Autodesk Inventor part; units mm, degrees
ref_plane "YZ Plane" through (0, 0, 0) normal (1, 0, 0) x (0, 1, 0)
ref_plane "XZ Plane" through (0, 0, 0) normal (0, 1, 0) x (-1, 0, 0)
ref_plane "XY Plane" through (0, 0, 0) normal (0, 0, 1) x (1, 0, 0)
sketch "스케치1" plane through (0, 0, 0) normal (0, 0, 1) x (1, 0, 0)
  line L0 (-28, 61.1) -> (28, 61.1)
  line L1 (28, 61.1) -> (28, -5.1)
  line L2 (28, -5.1) -> (-28, -5.1)
  line L3 (-28, -5.1) -> (-28, 61.1)
  point P0 (0, 0)
  dimension "d0" = 66.2
  dimension "d2" = 5.1
  dimension "d8" = 28
  dimension "d9" = 28
extrude "돌출1" add sketch "스케치1" along normal blind 4
sketch "스케치2" plane through (0, 0, 4) normal (0, 0, 1) x (1, 0, 0)
  line L0 (-2, 48) -> (-2, 6)
  line L1 (-32, 48) -> (-7.5, 48)
  line L2 (-2, 48) -> (4.5, 48)
  line L3 (16.5, 6) -> (16.5, 48)
  line L4 (10, 48) -> (16.5, 48)
  line L5 (10, 48) -> (10, 6)
  line L6 (10, 6) -> (16.5, 6)
  circle A0 centre (13, 45) radius 1.6
  circle A1 centre (13, 9) radius 1.6
  line L7 (28.5, 6) -> (28.5, 48)
  line L8 (22, 48) -> (28.5, 48)
  line L9 (22, 48) -> (22, 6)
  line L10 (22, 6) -> (28.5, 6)
  circle A2 centre (25, 45) radius 1.6
  circle A3 centre (25, 9) radius 1.6
  line L11 (-7.5, 6) -> (-7.5, 48)
  line L12 (-32, 48) -> (-7.5, 48)
  line L13 (-32, 48) -> (-32, 52)
  line L14 (-38, 52) -> (-32, 52)
  line L15 (-38, 2) -> (-38, 52)
  line L16 (-38, 2) -> (-32, 2)
  line L17 (-32, 2) -> (-32, 6)
  line L18 (-32, 6) -> (-7.5, 6)
  circle A4 centre (-35, 45) radius 1.6
  circle A5 centre (-35, 9) radius 1.6
  circle A6 centre (-23, 45) radius 1.6
  circle A7 centre (-23, 9) radius 1.6
  circle A8 centre (-11, 45) radius 1.6
  circle A9 centre (-11, 9) radius 1.6
  line L19 (-2, 6) -> (4.5, 6)
  circle A10 centre (1, 45) radius 1.6
  circle A11 centre (1, 9) radius 1.6
  line L20 (-2, 48) -> (0, 48)
  line L21 (0, 48) -> (0, 6)
  point P0 (0, 0)
  point P1 (-13, 26)
  dimension "d7" = 2
extrude "돌출2" cut sketch "스케치2" against normal up to surface (4 mm away) contours L21 A10 | A10 L21 | L21 A11 | A11 L21 | A0 | A1 | A2 | A3 | A6 | A7 | A8 | A9
sketch "스케치3" plane through (0, 0, 4) normal (0, 0, 1) x (1, 0, 0)
  circle A0 centre (-23, 45) radius 1.6
  circle A1 centre (-11, 45) radius 1.6
  circle A2 centre (-11, 9) radius 1.6
  circle A3 centre (25, 9) radius 1.6
  circle A4 centre (13, 45) radius 1.6
  circle A5 centre (1, 9) radius 1.6
  circle A6 centre (1, 45) radius 1.6
  circle A7 centre (13, 9) radius 1.6
  circle A8 centre (25, 45) radius 1.6
  circle A9 centre (-23, 9) radius 1.6
  line L0 (28, 61.1) -> (-28, 61.1)
  line L1 (-28, 61.1) -> (-28, -5.1)
  line L2 (-28, -5.1) -> (28, -5.1)
  line L3 (28, -5.1) -> (28, 61.1)
  line L4 (-23, 45) -> (-23, 9)
  line L5 (-23, 27) -> (-28, 27)
  line L6 (-28, -5.1) -> (-28, 61.1)
  circle A10 centre (-28, 27) radius 5
  point P0 (0, 0)
  dimension "d12" = 18
  dimension "d15" = 10
extrude "돌출3" cut sketch "스케치3" against normal blind 4 contours A10 L5 L1 | L1 A10 | L5 A10 L1
sketch "스케치4" plane through (0, 0, 4) normal (0, 0, 1) x (1, 0, 0)
  arc A0 (-28, 22) -> (-28, 32) centre (-28, 27) ccw
  line L0 (-28, 22) -> (-28, -5.1)
  line L1 (-28, -5.1) -> (28, -5.1)
  line L2 (28, -5.1) -> (28, 61.1)
  line L3 (28, 61.1) -> (-28, 61.1)
  line L4 (-28, 61.1) -> (-28, 32)
  circle A1 centre (-23, 9) radius 1.6
  circle A2 centre (25, 45) radius 1.6
  circle A3 centre (13, 9) radius 1.6
  circle A4 centre (1, 45) radius 1.6
  circle A5 centre (1, 9) radius 1.6
  circle A6 centre (13, 45) radius 1.6
  circle A7 centre (25, 9) radius 1.6
  circle A8 centre (-11, 9) radius 1.6
  circle A9 centre (-11, 45) radius 1.6
  circle A10 centre (-23, 45) radius 1.6
  circle A11 centre (-18, -2.6) radius 1.6
  circle A12 centre (-8, -2.6) radius 1.6
  circle A13 centre (8, -2.6) radius 1.6
  circle A14 centre (18, -2.6) radius 1.6
  point P0 (0, 0)
  dimension "d16" = 3.2
  dimension "d17" = 3.2
  dimension "d18" = 3.2
  dimension "d19" = 3.2
  dimension "d20" = 2.5
  dimension "d21" = 2.5
  dimension "d22" = 2.5
  dimension "d23" = 2.5
  dimension "d24" = 10
  dimension "d25" = 20
  dimension "d26" = 10
  dimension "d27" = 20
extrude "돌출4" cut sketch "스케치4" against normal up to surface (4 mm away) contours A11 | A12 | A13 | A14
sketch "스케치5" plane through (0, 0, 4) normal (0, 0, 1) x (1, 0, 0)
  circle A0 centre (8, -2.6) radius 1.6
  circle A1 centre (18, -2.6) radius 1.6
  circle A2 centre (-8, -2.6) radius 1.6
  circle A3 centre (-18, -2.6) radius 1.6
  arc A4 (-28, 22) -> (-28, 32) centre (-28, 27) ccw
  line L0 (-28, 22) -> (-28, -5.1)
  line L1 (-28, -5.1) -> (28, -5.1)
  line L2 (28, -5.1) -> (28, 61.1)
  line L3 (28, 61.1) -> (-28, 61.1)
  line L4 (-28, 61.1) -> (-28, 32)
  circle A5 centre (-23, 9) radius 1.6
  circle A6 centre (25, 45) radius 1.6
  circle A7 centre (13, 9) radius 1.6
  circle A8 centre (1, 45) radius 1.6
  circle A9 centre (1, 9) radius 1.6
  circle A10 centre (13, 45) radius 1.6
  circle A11 centre (25, 9) radius 1.6
  circle A12 centre (-11, 9) radius 1.6
  circle A13 centre (-11, 45) radius 1.6
  circle A14 centre (-23, 45) radius 1.6
  circle A15 centre (-18, 56.6) radius 1.6
  circle A16 centre (-8, 56.6) radius 1.6
  circle A17 centre (8, 56.6) radius 1.6
  circle A18 centre (18, 56.6) radius 1.6
  point P0 (0, 0)
  dimension "d30" = 3.2
  dimension "d31" = 3.2
  dimension "d32" = 3.2
  dimension "d33" = 3.2
  dimension "d34" = 4.5
  dimension "d35" = 4.5
  dimension "d36" = 4.5
  dimension "d37" = 4.5
  dimension "d38" = 10
  dimension "d39" = 20
  dimension "d40" = 10
  dimension "d41" = 20
extrude "돌출5" cut sketch "스케치5" against normal up to surface (4 mm away) contours A15 | A16 | A17 | A18
fillet "모깎기1" radius 3 1 edges at (-28, 61.1, 2)
chamfer "모따기1" distance 1.5 angle 45 8 edges at (-19.6, 56.6, 4) (-9.6, 56.6, 4) (6.4, 56.6, 4) (16.4, 56.6, 4) (-19.6, 56.6, 0) (-9.6, 56.6, 0) (6.4, 56.6, 0) (16.4, 56.6, 0)
chamfer "모따기2" distance 1.5 angle 45 10 edges at (23.4, 45, 4) (11.4, 45, 4) (-0.6, 45, 4) (-12.6, 45, 4) (-24.6, 45, 4) (-24.6, 9, 4) (-12.6, 9, 4) (-0.6, 9, 4) (11.4, 9, 4) (23.4, 9, 4)
properties part number "J1J2_Side" material "알루미늄 6061"
The listing builds one solid part. Answer for the finished solid, in the listing's coordinates (mm). Coordinates: 2 decimals unless noted, no trailing zeros. Loops run counter-clockwise (first coordinate to the right, second up) from the corner with the lowest first, then second, coordinate; pieces in that order, holes last. Notation, with made-up numbers: (36, 30) -> (64, 30) arc R15 ccw to (64, 55) -> close; hole circle Ø2 at (27, 4.25). An arc over 180 degrees is marked (long way). Answer in a Markdown table with one row per item. Add a question column.
1. The part is cut by section B-B, the plane x = 13. Write down the section's boundary in (y, z).
2. Flat-ended cylindrical pins translate along their axes: P1, Ø4, axis at x = -18, y = 56.6, coming from the +Z side; P2, Ø2, axis at x = 18, y = 27, coming from the -Z side; P3, Ø1.9, axis at x = -8, y = 56.6, coming from the +Z side; P4, Ø5, axis at x = -23, y = 9, coming from the +Z side. Find the tip coordinate at first contact, or state that the pin passes through.
3. Consider line 1 (Y direction, x = -11, z = 1.1); line 2 (Y direction, x = 8, z = 1.9); line 3 (X direction, y = 56.5, z = 3.85). Determine where each line is inside the solid, lowest interval first. Write a range as [from, to].
4. The part is cut by section C-C, the plane y = -2.6. Write down the section's boundary in (x, z), then the cut area to 3 significant figures.
5. Determine the mould class of faces 1 (the flat face through (-28, 8, 2)), 2 (the cylindrical face through (25.74, 43.58, 1.27)), 3 (the flat face through (1, 61.1, 2)) for opening direction Y: +Y half, -Y half, draft (parallel to the pull), parting line (faces both ways), or undercut.
6. The part is cut by section A-A, the plane y = 45. Count the separate pieces of the cut face and the enclosed holes in it, then the cut area to 3 significant figures.
Answer below:
| question | item | result |
|---|---|---|
| 1 | outline | (-5.1, 0) -> (7.4, 0) -> (7.4, 2.5) -> (5.9, 4) -> (-5.1, 4) -> close; (10.6, 0) -> (43.4, 0) -> (43.4, 2.5) -> (41.9, 4) -> (12.1, 4) -> (10.6, 2.5) -> close; (46.6, 0) -> (61.1, 0) -> (61.1, 4) -> (48.1, 4) -> (46.6, 2.5) -> close |
| 2 | P1 | z = 2.9 |
| 2 | P2 | z = 0 |
| 2 | P3 | through |
| 2 | P4 | z = 3.4 |
| 3 | line 1 | [-5.1, 7.4], [10.6, 43.4], [46.6, 61.1] |
| 3 | line 2 | [-5.1, -4.2], [-1, 55], [58.2, 61.1] |
| 3 | line 3 | [-28, -20.95], [-15.05, -10.95], [-5.05, 5.05], [10.95, 15.05], [20.95, 28] |
| 4 | outline | (-28, 0) -> (-19.6, 0) -> (-19.6, 4) -> (-28, 4) -> close; (-16.4, 0) -> (-9.6, 0) -> (-9.6, 4) -> (-16.4, 4) -> close; (-6.4, 0) -> (6.4, 0) -> (6.4, 4) -> (-6.4, 4) -> close; (9.6, 0) -> (16.4, 0) -> (16.4, 4) -> (9.6, 4) -> close; (19.6, 0) -> (28, 0) -> (28, 4) -> (19.6, 4) -> close |
| 4 | area | 173 mm2 |
| 5 | face 1 | draft |
| 5 | face 2 | undercut |
| 5 | face 3 | +Y half |
| 6 | separate pieces | 6 |
| 6 | enclosed holes | 0 |
| 6 | area | 149 mm2 |
